Read the model definition and answer for the solid it produces. Units are mm, in the model's axes. A direction names the side the tool comes from. Coordinates: 2 decimals unless noted, no trailing zeros. Order: outer loops, then holes, each group sorted by start corner. A loop starts at its lowest first (then second) coordinate and runs counter-clockwise, first axis right, second up. Notation, with made-up numbers: M 48.25,26.25 L 52.25,26.25 A18 cw 52.25,59.25 Z; hole C 25,-6 d1. An arc over 180 degrees is marked long. Use a Markdown table: item, result. Add a question column.
1) Find the intervals of material crossed by probe 1 along X at (y, z) = (6.75, 2.5); probe 2 along Z at (x, y) = (0.5, 14.5); probe 3 along Y at (x, z) = (0, 7.9), in increasing order. Write a range as [from, to].
2) Find section C-C on z = 3. Write down the section's boundary in (x, y), plus the area to 3 significant figures.
3) The mould has two halves that part along Z. Classify faces 6 (the face through (3, 8, 6.5)), 7 (the face through (-2, 10, -3)), 8 (the face through (5, 10, 0)), 9 (the face through (5, -2.7, 8)): released by +Z, released by -Z, zero draft, split by the parting line, or undercut.
4) Find section D-D on y = 15.66. Write down the section's boundary in (x, z).
5) Find section B-B on y = 0. Write down the section's boundary in (x, z).
6) Find section A-A on x = 10.39. Write down the section's boundary in (y, z), plus the area to 3 significant figures.
7) Each of these flat-tipped pins is pushed along its axis until it touches: pin 1 Ø2 at (x, y) = (0, 0) entering from +Z; pin 2 Ø2.5 at (x, z) = (-8, 3) entering from +Y; pin 3 Ø1.2 at (x, z) = (6, 8) entering from -Y; pin 4 Ø3 at (y, z) = (15.66, 3) entering from -X. Where does it stop, or does it pass through?
8) For faces 1 (the face through (11.545, -0.479, -1.479)), 2 (the face through (15.72, 7, 3)), 3 (the face through (2.425, -4, 8)), 4 (the face through (-21.49, 20.43, 4.5)), 5 (the face through (-9.78, 14.7, 4.4)), determine the directions among +Z, -Z, +X, -X, +Y, -Y from which every point of the face is accessible in a straight line to the end or side of a thin tool.
from build123d import *

# Parameters (mm, degrees)
SKETCH1_W              = 30
SKETCH1_H              = 24.4
BOSS_EXTRUDE1_DEPTH    = 3
SKETCH1_5_R            = 1.25
CUT_EXTRUDE1_DEPTH     = 6
BOSS_EXTRUDE3_START    = -3
BOSS_EXTRUDE3_DEPTH    = 3
SKETCH1_6_W            = 4.5
SKETCH1_6_H            = 11
SKETCH1_6_H_2          = 24.4
BOSS_EXTRUDE4_DEPTH    = 9
BOSS_EXTRUDE5_START    = -3
SKETCH2_6_W            = 14.75
SKETCH2_6_H            = 28.06
BOSS_EXTRUDE5_DEPTH    = 9
CUT_REVOLVE1_OUTLINE_W = 1.25
CUT_REVOLVE1_OUTLINE_H = 4.5
BOSS_EXTRUDE7_START    = 9
SKETCH1_7_W            = 2.25
SKETCH1_7_H            = 2
SKETCH1_7_W_2          = 6.505
SKETCH1_7_W_3          = 1.2
SKETCH1_7_W_4          = 6.495
SKETCH1_7_W_5          = 1.25
SKETCH1_7_R            = 1.25
BOSS_EXTRUDE7_DEPTH    = 2.5


# Read off the part's stored shape, not the designer's step: Cut-Revolve1
with BuildPart() as part:
    # Sketch1 → Boss-Extrude1 (new body)
    with BuildSketch(Plane.XY):
        with Locations((5.22, 7.5)):
            Rectangle(SKETCH1_W, SKETCH1_H)
    extrude(amount=-BOSS_EXTRUDE1_DEPTH)

    # Sketch1<5> → Cut-Extrude1 (cut)
    with BuildSketch(Plane.XY):
        Circle(SKETCH1_5_R)
        with Locations((10.39, 0)):
            Circle(SKETCH1_5_R)
    extrude(amount=-CUT_EXTRUDE1_DEPTH, mode=Mode.SUBTRACT)

    # Sketch2 → Boss-Extrude3 (add)
    with BuildSketch(Plane.XY.offset(3).offset(BOSS_EXTRUDE3_START)):
        Polygon((-9.78, -4.7), (-9.78, 16.91), (-4.78, 16.91), (-4.78, 19.7), (20.22, 19.7), (20.22, 23.36), (-24.53, 23.36), (-24.53, -4.7), align=None)
    extrude(amount=-BOSS_EXTRUDE3_DEPTH)

    # Sketch1<6> → Boss-Extrude4 (add)
    with BuildSketch(Plane.XY):
        with Locations((-7.53, 0.8)):
            Rectangle(SKETCH1_6_W, SKETCH1_6_H)
        with Locations((17.97, 7.5)):
            Rectangle(SKETCH1_6_W, SKETCH1_6_H_2)
    extrude(amount=BOSS_EXTRUDE4_DEPTH)

    # Sketch2<6> → Boss-Extrude5 (add)
    with BuildSketch(Plane.XY.offset(3).offset(BOSS_EXTRUDE5_START)):
        with Locations((-17.155, 9.33)):
            Rectangle(SKETCH2_6_W, SKETCH2_6_H)
    extrude(amount=BOSS_EXTRUDE5_DEPTH)

    # Cut-Revolve1 outline → Cut-Revolve1 (revolve, cut)
    with BuildSketch(Plane(origin=(0, 15.66, 3), x_dir=(0, 1, 0), z_dir=(0, 0, -1))):
        Polygon((5, -24.53), (5, -18.53), (1.25, -14.78), (1.25, -9.78), (0, -9.78), (0, -24.53), align=None)
        with Locations((0.625, 17.97)):
            Rectangle(CUT_REVOLVE1_OUTLINE_W, CUT_REVOLVE1_OUTLINE_H)
    revolve(axis=Axis((0, 15.66, 3), (1, 0, 0)), mode=Mode.SUBTRACT)

    # Sketch1<7> → Boss-Extrude7 (add)
    # profile 1 of 9: a face of its own
    with BuildSketch(Plane.XY.offset(BOSS_EXTRUDE7_START)):
        Polygon((-9.78, 19.7), (-9.78, 9.7), (13.47, 9.7), (15.72, 9.7), (15.72, 19.7), align=None)
    # profile 2 of 9: a face of its own
    with BuildSketch(Plane.XY.offset(BOSS_EXTRUDE7_START)):
        Polygon((13.47, 9.7), (-9.78, 9.7), (-9.78, 7.8), (-5.28, 7.8), (-5.28, 7.4), (-5.28, -2.7), (15.72, -2.7), (15.72, 7.7), (13.47, 7.7), align=None)
        with BuildLine():
            Line((-5.08, -2), (-5.08, 6.2))
            ThreePointArc((-5.08, 6.2), (-4.787106781, 6.907106781), (-4.08, 7.2))
            Line((-4.08, 7.2), (3.92, 7.2))
            Line((3.92, 7.2), (3.92, 7.5))
            Line((3.92, 7.5), (14.47, 7.5))
            ThreePointArc((14.47, 7.5), (15.177106781, 7.207106781), (15.47, 6.5))
            Line((15.47, 6.5), (15.47, -2))
            ThreePointArc((15.47, -2), (15.323553391, -2.353553391), (14.97, -2.5))
            Line((14.97, -2.5), (-4.58, -2.5))
            ThreePointArc((-4.58, -2.5), (-4.933553391, -2.353553391), (-5.08, -2))
        make_face(mode=Mode.SUBTRACT)
    # profile 3 of 9: a face of its own
    with BuildSketch(Plane.XY.offset(BOSS_EXTRUDE7_START)):
        Polygon((-5.28, 6.3), (-5.28, 7.4), (-5.28, 7.8), (-9.78, 7.8), (-9.78, 6.3), align=None)
    # profile 4 of 9: a face of its own
    with BuildSketch(Plane.XY.offset(BOSS_EXTRUDE7_START)):
        with Locations((14.595, 8.7)):
            Rectangle(SKETCH1_7_W, SKETCH1_7_H)
    # profile 5 of 9: a face of its own
    with BuildSketch(Plane.XY.offset(BOSS_EXTRUDE7_START)):
        with Locations((-0.8275, -3.7)):
            Rectangle(SKETCH1_7_W_2, SKETCH1_7_H)
    # profile 6 of 9: a face of its own
    with BuildSketch(Plane.XY.offset(BOSS_EXTRUDE7_START)):
        with Locations((-4.68, -3.7)):
            Rectangle(SKETCH1_7_W_3, SKETCH1_7_H)
    # profile 7 of 9: a face of its own
    with BuildSketch(Plane.XY.offset(BOSS_EXTRUDE7_START)):
        with Locations((11.2225, -3.7)):
            Rectangle(SKETCH1_7_W_4, SKETCH1_7_H)
    # profile 8 of 9: a face of its own
    with BuildSketch(Plane.XY.offset(BOSS_EXTRUDE7_START)):
        with Locations((15.095, -3.7)):
            Rectangle(SKETCH1_7_W_5, SKETCH1_7_H)
    # profile 9 of 9: a face of its own
    with BuildSketch(Plane.XY.offset(BOSS_EXTRUDE7_START)):
        with BuildLine():
            ThreePointArc((-5.08, 6.2), (-4.787106781, 6.907106781), (-4.08, 7.2))
            Line((-4.08, 7.2), (3.92, 7.2))
            Line((3.92, 7.2), (3.92, 7.5))
            Line((3.92, 7.5), (14.47, 7.5))
            ThreePointArc((14.47, 7.5), (15.177106781, 7.207106781), (15.47, 6.5))
            Line((15.47, 6.5), (15.47, -2))
            ThreePointArc((15.47, -2), (15.323553391, -2.353553391), (14.97, -2.5))
            Line((14.97, -2.5), (-4.58, -2.5))
            ThreePointArc((-4.58, -2.5), (-4.933553391, -2.353553391), (-5.08, -2))
            Line((-5.08, -2), (-5.08, 6.2))
        make_face()
        with Locations((10.39, 0)):
            Circle(SKETCH1_7_R, mode=Mode.SUBTRACT)
        Circle(SKETCH1_7_R, mode=Mode.SUBTRACT)
    extrude(amount=-BOSS_EXTRUDE7_DEPTH)


solid = part.part
Check result:
| question | item | result |
|---|---|---|
| 1 | probe 1 | x = [-24.53, -9.78], [15.72, 20.22] |
| 1 | probe 2 | z = [-3, 0], [6.5, 9] |
| 1 | probe 3 | y = [-4.7, -1.25], [1.25, 19.7] |
| 2 | outline | M -24.53,-4.7 L -5.28,-4.7 L -5.28,6.3 L -9.78,6.3 L -9.78,14.41 L -14.78,14.41 L -18.53,10.66 L -24.53,10.66 Z; M -24.53,20.66 L -18.53,20.66 L -14.78,16.91 L -9.78,16.91 L -9.78,23.36 L -24.53,23.36 Z; M 15.72,-4.7 L 20.22,-4.7 L 20.22,14.41 L 15.72,14.41 Z; M 15.72,16.91 L 20.22,16.91 L 20.22,19.7 L 15.72,19.7 Z |
| 2 | area | 466 mm2 |
| 3 | face 6 | undercut |
| 3 | face 7 | released by -Z |
| 3 | face 8 | undercut |
| 3 | face 9 | zero draft |
| 4 | outline | M -24.53,-3 L 20.22,-3 L 20.22,1.75 L 15.72,1.75 L 15.72,0 L -9.78,0 L -9.78,1.75 L -14.78,1.75 L -18.53,-2 L -24.53,-2 Z; M -24.53,8 L -18.53,8 L -14.78,4.25 L -9.78,4.25 L -9.78,6.5 L 15.72,6.5 L 15.72,4.25 L 20.22,4.25 L 20.22,9 L -24.53,9 Z |
| 5 | outline | M -24.53,-3 L -1.25,-3 L -1.25,0 L -5.28,0 L -5.28,6.5 L -1.25,6.5 L -1.25,9 L -24.53,9 Z; M 1.25,-3 L 9.14,-3 L 9.14,0 L 1.25,0 Z; M 1.25,6.5 L 9.14,6.5 L 9.14,9 L 1.25,9 Z; M 11.64,-3 L 20.22,-3 L 20.22,9 L 11.64,9 L 11.64,6.5 L 15.72,6.5 L 15.72,0 L 11.64,0 Z |
| 6 | outline | M -4.7,-3 L -1.25,-3 L -1.25,0 L -4.7,0 Z; M -4.7,6.5 L -1.25,6.5 L -1.25,9 L -4.7,9 Z; M 1.25,-3 L 23.36,-3 L 23.36,0 L 1.25,0 Z; M 1.25,6.5 L 19.7,6.5 L 19.7,9 L 1.25,9 Z |
| 6 | area | 131 mm2 |
| 7 | pin 1 | passes through |
| 7 | pin 2 | stops at y = 6.3 |
| 7 | pin 3 | stops at y = -2.7 |
| 7 | pin 4 | stops at x = -15.03 |
| 8 | face 1 | +Z, -Z |
| 8 | face 2 | +Y, -Y |
| 8 | face 3 | +Z, -Y |
| 8 | face 4 | -X |
| 8 | face 5 | +Y |
